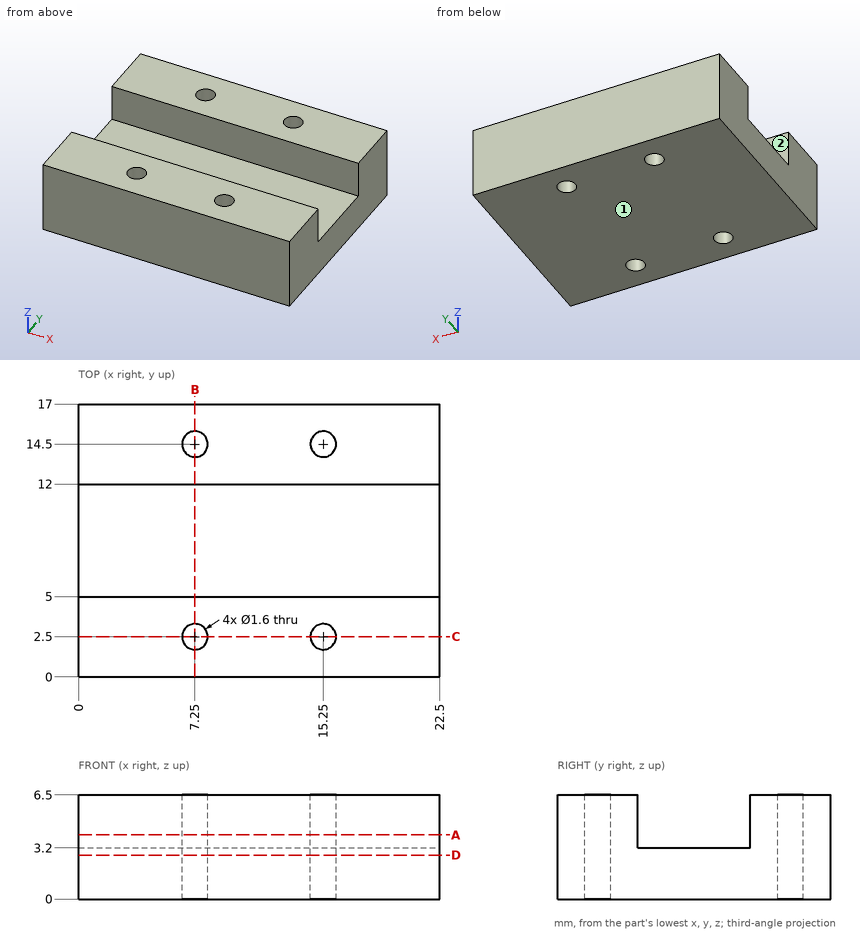
Part print with two shaded views. Sizes in mm from the minimum x, y, z corner. A direction names the side the tool comes from. Round coordinates to 2 decimals unless told otherwise and drop trailing zeros. Order: outer loops, then holes, each group sorted by start corner. A loop starts at its lowest first (then second) coordinate and runs counter-clockwise, first axis right, second up.
(1) Band-saw the part on D-D (z = 2.75). List the corners of the cut face in (x, y), then the cut area to 3 significant figures.
(2) Band-saw the part on B-B (x = 7.25). List the corners of the cut face in (y, z).
(3) 3-axis set-ups, long thin cutter, end or side, ignore diameter. For the marked faces 1 and 2: which of +Z, -Z, +X, -X, +Y, -Y reach the whole face in a straight line?
(4) Band-saw the part on A-A (z = 4). List the corners of the cut face in (x, y), then the cut area to 3 significant figures.
(5) Band-saw the part on C-C (y = 2.5). List the corners of the cut face in (x, z), then the cut area to 3 significant figures.
(6) Pin check, flat tip, straight feed: pin 1 (2 mm diameter, centred on x = 14, y = 9, fed in from +Z). Stop position of the tip, or through.
(7) Drill centre lines: line 1 (Y direction, x = 7.25, z = 2.25); line 2 (Y direction, x = 7.25, z = 3.5); line 3 (Y direction, x = 19.25, z = 3.5). Where is each one in solid material? Low to high.
Verdict:
1. outline: (0, 0) - (22.5, 0) - (22.5, 17) - (0, 17) - close; hole circle Ø1.6 at (7.25, 2.5); hole circle Ø1.6 at (7.25, 14.5); hole circle Ø1.6 at (15.25, 2.5); hole circle Ø1.6 at (15.25, 14.5)
1. area: 374 mm2
2. outline: (0, 0) - (1.7, 0) - (1.7, 6.5) - (0, 6.5) - close; (3.3, 0) - (13.7, 0) - (13.7, 6.5) - (12, 6.5) - (12, 3.2) - (5, 3.2) - (5, 6.5) - (3.3, 6.5) - close; (15.3, 0) - (17, 0) - (17, 6.5) - (15.3, 6.5) - close
3. face 1: -Z, +X, -X, +Y, -Y
3. face 2: +Z, +X, -X
4. outline: (0, 0) - (22.5, 0) - (22.5, 5) - (0, 5) - close; (0, 12) - (22.5, 12) - (22.5, 17) - (0, 17) - close; hole circle Ø1.6 at (7.25, 2.5); hole circle Ø1.6 at (7.25, 14.5); hole circle Ø1.6 at (15.25, 2.5); hole circle Ø1.6 at (15.25, 14.5)
4. area: 217 mm2
5. outline: (0, 0) - (6.45, 0) - (6.45, 6.5) - (0, 6.5) - close; (8.05, 0) - (14.45, 0) - (14.45, 6.5) - (8.05, 6.5) - close; (16.05, 0) - (22.5, 0) - (22.5, 6.5) - (16.05, 6.5) - close
5. area: 125 mm2
6. pin 1: stops at z = 3.2
7. line 1: y = 0 to 1.7, 3.3 to 13.7, 15.3 to 17
7. line 2: y = 0 to 1.7, 3.3 to 5, 12 to 13.7, 15.3 to 17
7. line 3: y = 0 to 5, 12 to 17
